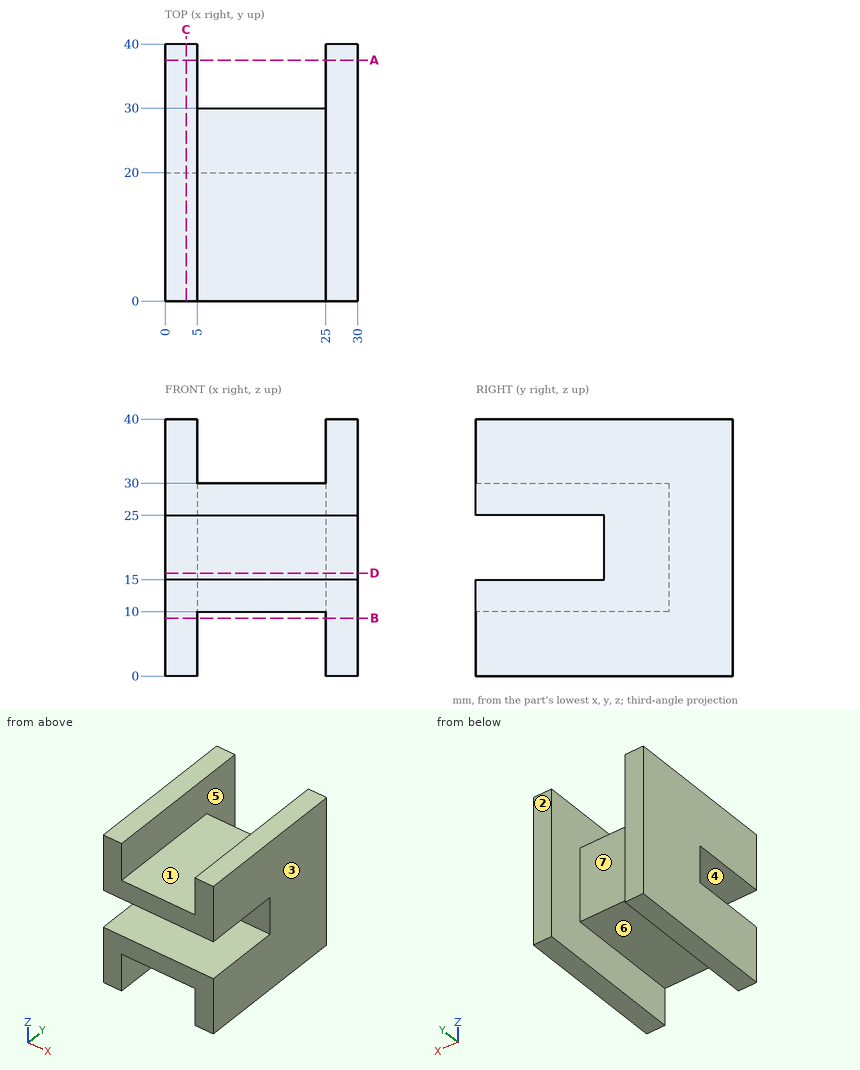
Print and shaded views of the part. All mm, measured from the part's lowest x, y and z. A direction names the side the tool comes from. Give positions to 0.01 mm unless a question says otherwise; leave off trailing zeros. Loops run counter-clockwise (first coordinate to the right, second up) from the corner with the lowest first, then second, coordinate; pieces in that order, holes last.
1) Saw through at C-C (x = 3.25). Write the cut outline in (y, z), plus the area to 3 significant figures.
2) Flat gauge pins, fed straight in: pin 1 Ø6 at (x, y) = (19, 32.5) entering from -Z; pin 2 Ø3 at (x, y) = (7, 9.5) entering from +Z; pin 3 Ø16 at (x, z) = (19.5, 23.5) entering from +Y; pin 4 Ø5 at (x, z) = (11, 18) entering from -Y. Where does each tip first touch, or does it go through?
3) Pull direction X, two halves, no side cores. Call the marked faces 1, 2 and 3: +X half, -X half, draft (parallel to the pull), parting line (faces both ways), or undercut.
4) Tool access for the marked faces 4, 5, 6 and 7: list every direction of +Z, -Z, +X, -X, +Y, -Y with a clear straight run to the whole face (end or side of a thin tool).
5) Saw through at D-D (z = 16). Write the cut outline in (x, y), plus the area to 3 significant figures.
6) Wall check: line 1 (X direction, y = 23, z = 4); line 2 (Z direction, x = 23.5, y = 10); line 3 (Z direction, x = 28.5, y = 14). Give the ranges that are in metal, low to high.
7) Saw through at A-A (y = 37.5). Write the cut outline in (x, z).
Answer block:
1. outline: (0, 0) - (40, 0) - (40, 40) - (0, 40) - (0, 25) - (20, 25) - (20, 15) - (0, 15) - close
1. area: 1,400 mm2
2. pin 1: stops at z = 10
2. pin 2: stops at z = 30
2. pin 3: stops at y = 40
2. pin 4: stops at y = 20
3. face 1: undercut
3. face 2: draft
3. face 3: +X half
4. face 4: +X, -X, -Y
4. face 5: +Y
4. face 6: -Z, +Y, -Y
4. face 7: +Z, -Z, +Y
5. outline: (0, 20) - (30, 20) - (30, 40) - (25, 40) - (25, 30) - (5, 30) - (5, 40) - (0, 40) - close
5. area: 400 mm2
6. line 1: x = 0 to 5, 25 to 30
6. line 2: z = 10 to 15, 25 to 30
6. line 3: z = 0 to 15, 25 to 40
7. outline: (0, 0) - (5, 0) - (5, 40) - (0, 40) - close; (25, 0) - (30, 0) - (30, 40) - (25, 40) - close
